Part model, mm, in its own coordinate system. Face numbers are marked on the shaded views. A direction names the side the tool comes from. Round coordinates to 2 decimals unless told otherwise and drop trailing zeros. Loops run counter-clockwise (first coordinate to the right, second up) from the corner with the lowest first, then second, coordinate; pieces in that order, holes last.
1) Band-saw the part on D-D, the plane y = 3.25. Write the cut outline in (x, z).
2) Band-saw the part on B-B, the plane y = 7. Write the cut outline in (x, z), then the cut area to 3 significant figures.
3) Probe line 1 (X direction, y = 5.5, z = 0); line 2 (Y direction, x = -3, z = 6); line 3 (X direction, y = 1.5, z = -5.5). List the from-to ranges inside material, lowest first.
4) Band-saw the part on A-A, the plane x = 0. Write the cut outline in (y, z).
5) Band-saw the part on C-C, the plane z = 0. Write the cut outline in (x, y), then the cut area to 3 significant figures.
6) 3-axis set-ups, long thin cutter, end or side, ignore diameter. For the marked faces 1 and 2: which of +Z, -Z, +X, -X, +Y, -Y reach the whole face in a straight line?
7) Drop flat-ended pins along their axis: P1, Ø2.5, axis at x = 0, y = 6, coming from the -Z side (3 decimals); P2, Ø1, axis at x = 2.5, y = 5.5, coming from the +Z side; P3, Ø4, axis at y = 2.5, z = -4.5, coming from the +X side; P4, Ø5, axis at x = 0, z = 0, coming from the +Y side. Give the stop position or say it passes through.
8) Mould opens along X. For the marked faces 3, 4 and 5 say: +X half, -X half, draft (parallel to the pull), parting line (faces both ways), or undercut.
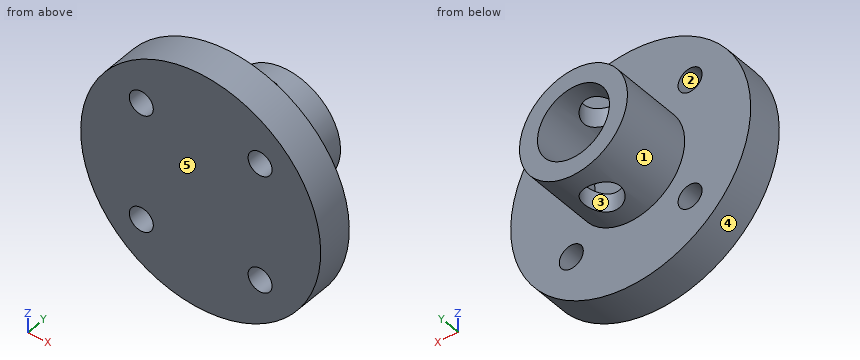
from build123d import *

# Parameters (mm, degrees)
CROQUIS1_R                 = 10
CROQUIS1_R_2               = 1
SALIENTE_EXTRUIR1_DEPTH    = 3
SALIENTE_EXTRUIR2_START    = 3
CROQUIS1_3_R               = 4.5
CROQUIS1_3_R_2             = 3
SALIENTE_EXTRUIR2_DEPTH    = 6
CORTAR_EXTRUIR1_DEPTH      = 17.763054614
CORTAR_EXTRUIR1_DEPTH_BACK = 17.763054614
CROQUIS2_R                 = 1.5


with BuildPart() as part:
    # Croquis1 → Saliente-Extruir1 (new body)
    with BuildSketch(Plane(origin=(0, 0, 0), x_dir=(1, 0, 0), z_dir=(0, 1, 0))):
        with Locations(Location((0, 0, 0), (0, 0, 270))):
            Circle(CROQUIS1_R)
        with Locations(Location((-4.949747468, 4.949747468, 0), (0, 0, 270))):
            Circle(CROQUIS1_R_2, mode=Mode.SUBTRACT)
        with Locations(Location((4.949747468, 4.949747468, 0), (0, 0, 270))):
            Circle(CROQUIS1_R_2, mode=Mode.SUBTRACT)
        with Locations(Location((4.949747468, -4.949747468, 0), (0, 0, 270))):
            Circle(CROQUIS1_R_2, mode=Mode.SUBTRACT)
        with Locations(Location((-4.949747468, -4.949747468, 0), (0, 0, 270))):
            Circle(CROQUIS1_R_2, mode=Mode.SUBTRACT)
    extrude(amount=SALIENTE_EXTRUIR1_DEPTH)

    # Croquis1<3> → Saliente-Extruir2 (add)
    with BuildSketch(Plane(origin=(0, 0, 0), x_dir=(1, 0, 0), z_dir=(0, 1, 0)).offset(SALIENTE_EXTRUIR2_START)):
        with Locations(Location((0, 0, 0), (0, 0, 270))):
            Circle(CROQUIS1_3_R)
        with Locations(Location((0, 0, 0), (0, 0, 270))):
            Circle(CROQUIS1_3_R_2, mode=Mode.SUBTRACT)
    extrude(amount=SALIENTE_EXTRUIR2_DEPTH)

    # Croquis2 → Cortar-Extruir1 (cut, two sides: drawn at the far end of the back side and taken through both)
    with BuildSketch(Plane.XY.offset(-CORTAR_EXTRUIR1_DEPTH_BACK)):
        with Locations((0, 6)):
            Circle(CROQUIS2_R)
    extrude(amount=CORTAR_EXTRUIR1_DEPTH + CORTAR_EXTRUIR1_DEPTH_BACK, mode=Mode.SUBTRACT)


solid = part.part
Reported:
1. outline: circle Ø9 at (0, 0); hole circle Ø6 at (0, 0)
2. outline: (-1.12, -4.36) - (-1.12, -2.78) arc R3 cw to (-1.12, 2.78) - (-1.12, 4.36) arc R4.5 ccw to start; (1.12, -4.36) arc R4.5 ccw to (1.12, 4.36) - (1.12, 2.78) arc R3 cw to (1.12, -2.78) - close
2. area: 28.5 mm2
3. line 1: x = -4.5 to -3, 3 to 4.5
3. line 2: y = 0 to 3
3. line 3: x = -8.35 to -5.78, -4.11 to 4.11, 5.78 to 8.35
4. outline: (0, -10) - (3, -10) - (3, -4.5) - (4.5, -4.5) - (4.5, -3) - (3, -3) - (3, 3) - (4.5, 3) - (4.5, 4.5) - (3, 4.5) - (3, 10) - (0, 10) - close; (7.5, -4.5) - (9, -4.5) - (9, -3) - (7.5, -3) - close; (7.5, 3) - (9, 3) - (9, 4.5) - (7.5, 4.5) - close
5. outline: (-10, 0) - (10, 0) - (10, 3) - (4.5, 3) - (4.5, 9) - (3, 9) - (3, 3) - (-3, 3) - (-3, 9) - (-4.5, 9) - (-4.5, 3) - (-10, 3) - close
5. area: 78.0 mm2
6. face 1: +Y
6. face 2: +Y, -Y
7. P1: passes through
7. P2: stops at z = 4.03
7. P3: stops at x = 9.68
7. P4: stops at y = 3
8. face 3: undercut
8. face 4: parting line
8. face 5: draft
